Input: dimensioned drawing with shaded views. Units: mm. Origin: part minimum x, y, z. Coordinates: 2 decimals unless noted, no trailing zeros. Loops run counter-clockwise (first coordinate to the right, second up) from the corner with the lowest first, then second, coordinate; pieces in that order, holes last.
Item 1: Pull-direction query (Y, two-part tool) for the marked faces 1, 2 and 3; classes: released by +Y, released by -Y, zero draft, split by the parting line, or undercut.
Item 2: Contact query for flat-ended pins moving along their axis: P1, Ø3, axis at y = 3.5, z = 7.5, coming from the -X side; P2, Ø0.7, axis at x = 3, y = 3, coming from the -Z side; P3, Ø2, axis at x = 5, z = 11, coming from the -Y side. Output: stop coordinate, or through.
Item 3: Section B-B on z = 4.75. Return loops of the section in (x, y).
Item 4: Ray query, line 1 along Z through (x, y) = (4.2, 0.75); line 2 along Y through (x, z) = (2.35, 3.25) (1 decimal); line 3 along Z through (x, y) = (1.2, 0.6) (1 decimal). Return the intervals inside material, ascending.
Item 5: Section A-A on z = 1.75. Return loops of the section in (x, y).
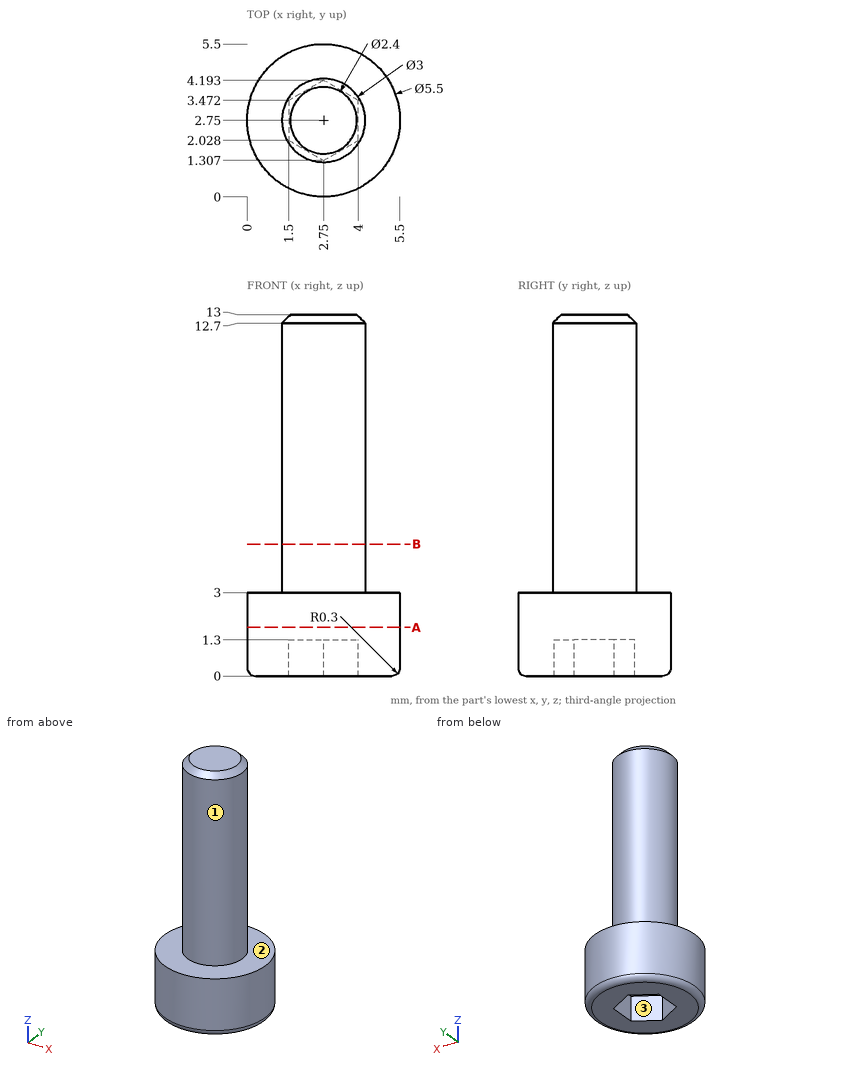
Results found:
1. face 1: split by the parting line
1. face 2: zero draft
1. face 3: undercut
2. P1: stops at x = 1.25
2. P2: stops at z = 1.3
2. P3: stops at y = 1.92
3. outline: circle Ø3 at (2.75, 2.75)
4. line 1: z = 0 to 3
4. line 2: y = 1.3 to 4.2
4. line 3: z = 0.1 to 3
5. outline: circle Ø5.5 at (2.75, 2.75)
